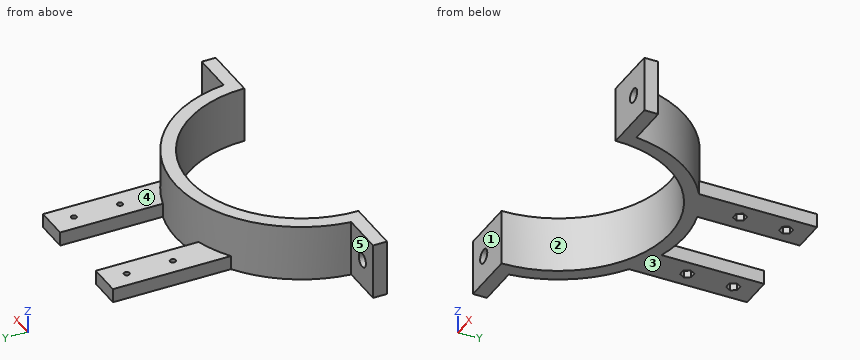
from build123d import *

# Parameters (mm, degrees)
BOSS_EXTRUDE1_DEPTH = 20
F_3DSKETCH3_R       = 1
BOSS_EXTRUDE2_DEPTH = 5
CUT_EXTRUDE1_DEPTH  = 2.5
SKETCH3_R           = 2.5
CUT_EXTRUDE2_DEPTH  = 99.107084352


with BuildPart() as part:
    # Sketch1 → Boss-Extrude1 (new body)
    with BuildSketch(Plane.XY):
        with BuildLine():
            Line((-45, 0), (-40, 0))
            ThreePointArc((-40, 0), (0, 40), (40, 0))
            Line((40, 0), (45, 0))
            Line((45, 0), (60, 0))
            Line((60, 0), (60, 5))
            Line((60, 5), (44.72135955, 5))
            ThreePointArc((44.72135955, 5), (0, 45), (-44.72135955, 5))
            Line((-44.72135955, 5), (-60, 5))
            Line((-60, 5), (-60, 0))
            Line((-60, 0), (-45, 0))
        make_face()
    extrude(amount=BOSS_EXTRUDE1_DEPTH)

    # 3DSketch3 → Boss-Extrude2 (add)
    with BuildSketch(Plane(origin=(-24.5, 37.7458607, 0), x_dir=(0.7573108303632157, 0.6530545966568009, 0), z_dir=(0, 0, -1))):
        with BuildLine():
            Line((0, 0), (27.594259898, -31.999517319))
            Line((27.594259898, -31.999517319), (36.681989862, -24.16286216))
            Line((36.681989862, -24.16286216), (12.668546171, 3.684183209))
            ThreePointArc((12.668546171, 3.684183209), (6.470025326, 1.375289757), (0, 0))
        make_face()
        with Locations(Location((26.913688106, -22.022703097, 0), (0, 0, 40.772303251))):
            Circle(F_3DSKETCH3_R, mode=Mode.SUBTRACT)
        with Locations(Location((16.138287262, -9.527074396, 0), (0, 0, 40.772303251))):
            Circle(F_3DSKETCH3_R, mode=Mode.SUBTRACT)
        with BuildLine():
            Line((31.60131693, 20.010548126), (55.614760621, -7.836497243))
            Line((55.614760621, -7.836497243), (64.702307458, 0))
            Line((64.702307458, 0), (37.10815006, 31.999398456))
            ThreePointArc((37.10815006, 31.999398456), (34.796480727, 25.802065738), (31.60131693, 20.010548126))
        make_face()
        with Locations(Location((54.93418883, 2.14031698, 0), (0, 0, 40.772303251))):
            Circle(F_3DSKETCH3_R, mode=Mode.SUBTRACT)
        with Locations(Location((44.158787985, 14.635945681, 0), (0, 0, 40.772303251))):
            Circle(F_3DSKETCH3_R, mode=Mode.SUBTRACT)
    extrude(amount=-BOSS_EXTRUDE2_DEPTH)

    # Sketch2 → Cut-Extrude1 (cut)
    with BuildSketch(Plane(origin=(0, 0, 0), x_dir=(-1, 0, 0), z_dir=(0, 0, -1))):
        Polygon((-16.19, 55.5), (-17.345, 57.500518683), (-19.655, 57.500518683), (-20.81, 55.5), (-19.655, 53.499481317), (-17.345, 53.499481317), align=None)
        Polygon((-16.19, 72), (-17.345, 74.000518683), (-19.655, 74.000518683), (-20.81, 72), (-19.655, 69.999481317), (-17.345, 69.999481317), align=None)
        Polygon((20.81, 72), (19.655, 74.000518683), (17.345, 74.000518683), (16.19, 72), (17.345, 69.999481317), (19.655, 69.999481317), align=None)
        Polygon((20.81, 55.5), (19.655, 57.500518683), (17.345, 57.500518683), (16.19, 55.5), (17.345, 53.499481317), (19.655, 53.499481317), align=None)
    extrude(amount=-CUT_EXTRUDE1_DEPTH, mode=Mode.SUBTRACT)

    # Sketch3 → Cut-Extrude2 (cut, through all)
    with BuildSketch(Plane(origin=(0, 5, 0), x_dir=(1, 0, 0), z_dir=(0, 1, 0))):
        with Locations(Location((-52.5, -10, 0), (0, 0, 270))):
            Circle(SKETCH3_R)
        with Locations(Location((52.5, -10, 0), (0, 0, 270))):
            Circle(SKETCH3_R)
    extrude(amount=-CUT_EXTRUDE2_DEPTH, mode=Mode.SUBTRACT)


solid = part.part
The model under review builds one solid part; all positions refer to its coordinate system, in mm. Face numbers are marked on the shaded views. A direction names the side the tool comes from. Coordinates: 2 decimals unless noted, no trailing zeros. Loops run counter-clockwise (first coordinate to the right, second up) from the corner with the lowest first, then second, coordinate; pieces in that order, holes last. Notation, with made-up numbers: (7, 59.5) -> (46, 59.5) arc R18 cw to (46, 75.5) -> close; hole circle Ø7 at (69, 77.25). An arc over 180 degrees is marked (long way). Use a Markdown table: item, result. Add a question column.
1. Add section D-D on z = 17.5. Write out the cut boundary in (x, y), plus the area to 3 significant figures.
2. Draft analysis for pull direction X (two halves, no side actions). For the marked faces 1 and 2, state which applies: pulls with the +X half, pulls with the -X half, needs draft (parallel to the pull), parting line crosses it, or undercut.
3. Clearance check with flat-ended pins moving along their axes: pin 1 Ø8 at (x, y) = (-30, 45.5) entering from -Z; pin 2 Ø1.5 at (x, z) = (-47.5, 17) entering from -Y; pin 3 Ø2.5 at (y, z) = (66, 3.5) entering from +X; pin 4 Ø0.7 at (x, z) = (18, 0.5) entering from -Y. State where each tip first meets the part, or that it passes through.
4. To check wall thickness, follow line 1 (X direction, y = 72, z = 3.1); line 2 (X direction, y = 2.75, z = 10); line 3 (X direction, y = 75.5, z = 2.75). State the ranges of each line that lie inside material, in increasing order.
5. Add section C-C on z = 10. Write out the cut boundary in (x, y).
6. Machinability: for the marked faces 3, 4 and 5, which of the approach directions +Z, -Z, +X, -X, +Y, -Y give a long, thin tool a straight path to every point of the face, cutting with its end or side? Answer none if there is none.
7. Add section A-A on x = -52.5. Write out the cut boundary in (y, z), plus the area to 3 significant figures.
8. Add section B-B on y = 68. Write out the cut boundary in (x, z).
Returned:
| question | item | result |
|---|---|---|
| 1 | outline | (-60, 0) -> (-40, 0) arc R40 cw to (40, 0) -> (60, 0) -> (60, 5) -> (44.72, 5) arc R45 ccw to (-44.72, 5) -> (-60, 5) -> close |
| 1 | area | 819 mm² |
| 2 | face 1 | needs draft |
| 2 | face 2 | undercut |
| 3 | pin 1 | passes through |
| 3 | pin 2 | stops at y = 0 |
| 3 | pin 3 | stops at x = 24.5 |
| 3 | pin 4 | stops at y = 35.54 |
| 4 | line 1 | x = -24.5 to -19.5, -17.5 to -12.5, 12.5 to 17.5, 19.5 to 24.5 |
| 4 | line 2 | x = -60 to -55, -50 to -39.91, 39.91 to 50, 55 to 60 |
| 4 | line 3 | x = -24.5 to -12.5, 12.5 to 24.5 |
| 5 | outline | (-60, 0) -> (-55, 0) -> (-55, 5) -> (-60, 5) -> close; (-50, 0) -> (-40, 0) arc R40 cw to (40, 0) -> (50, 0) -> (50, 5) -> (44.72, 5) arc R45 ccw to (-44.72, 5) -> (-50, 5) -> close; (55, 0) -> (60, 0) -> (60, 5) -> (55, 5) -> close |
| 6 | face 3 | -Z, +X, -X, +Y, -Y |
| 6 | face 4 | +Z, +X, +Y |
| 6 | face 5 | +Z, -Z, -X, +Y |
| 7 | outline | (0, 0) -> (5, 0) -> (5, 7.5) -> (0, 7.5) -> close; (0, 12.5) -> (5, 12.5) -> (5, 20) -> (0, 20) -> close |
| 7 | area | 75.0 mm² |
| 8 | outline | (-24.5, 0) -> (-12.5, 0) -> (-12.5, 5) -> (-24.5, 5) -> close; (12.5, 0) -> (24.5, 0) -> (24.5, 5) -> (12.5, 5) -> close |
